For this review, take the finished solid that the model builds, in its own axes (mm). A direction names the side the tool comes from. Coordinates: 2 decimals unless noted, no trailing zeros. Loops run counter-clockwise (first coordinate to the right, second up) from the corner with the lowest first, then second, coordinate; pieces in that order, holes last. Notation, with made-up numbers: (11, -37) -> (34, -37) arc R15 cw to (34, -15) -> close; hole circle Ø5 at (-18, 12.25). An arc over 180 degrees is marked (long way). Answer in a Markdown table with one row per item.
Autodesk Inventor part; units mm, degrees
ref_plane "YZ Plane" through (0, 0, 0) normal (1, 0, 0) x (0, 1, 0)
ref_plane "XZ Plane" through (0, 0, 0) normal (0, 1, 0) x (-1, 0, 0)
ref_plane "XY Plane" through (0, 0, 0) normal (0, 0, 1) x (1, 0, 0)
sketch "Sketch1" plane through (0, 0, 0) normal (0, 0, 1) x (1, 0, 0)
  arc A0 (4.25, 0) -> (-4.25, 0) centre (0, 0) ccw
  line L0 (-18.2, 0) -> (18.2, 0)
  line L1 (-13, 0) -> (-13, 5.25)
  line L2 (-13, 5.25) -> (13, 5.25)
  line L3 (13, 5.25) -> (13, 0)
  line L4 (-13, 0) -> (-4.25, 0)
  line L5 (4.25, 0) -> (13, 0)
  dimension "d0" = 8.5
  dimension "d1" = 1
  dimension "d2" = 13
  dimension "d3" = 13
extrude "Extrusion1" add sketch "Sketch1" along normal blind 20 contours A0 L0 L1 L2 L3
sketch "Sketch2" plane through (-13, 5.25, 0) normal (0, 1, 0) x (1, 0, 0)
  line L0 (-4.8106, -10) -> (24.391, -10) construction
  line L1 (26, 0) -> (0, 0) construction
  line L2 (26, -20) -> (0, -20) construction
  circle A0 centre (5, -10) radius 2.4
  circle A1 centre (21, -10) radius 2.4
  point P0 (13, 0)
  dimension "d7" = 20
  dimension "d8" = 10
  dimension "d9" = 4.8
  dimension "d10" = 4.8
  dimension "d11" = 16
  dimension "d12" = 8
extrude "Extrusion2" cut sketch "Sketch2" against normal through all
sketch "Sketch3" plane through (-13, 0, 0) normal (0, -1, 0) x (1, 0, 0)
  line L0 (0, 0) -> (0, 20)
  line L1 (0, 2) -> (2, 2)
  line L2 (2, 2) -> (2, 18)
  line L3 (2, 18) -> (0, 18)
  line L4 (0, 18) -> (0, 2)
  line L5 (26, 0) -> (26, 20)
  line L6 (26, 2) -> (24, 2)
  line L7 (24, 2) -> (24, 18)
  line L8 (24, 18) -> (26, 18)
  line L9 (26, 18) -> (26, 2)
  line L10 (0, 0) -> (8.75, 0)
  line L11 (0, 20) -> (8.75, 20)
  line L12 (17.25, 20) -> (26, 20)
  line L13 (17.25, 0) -> (26, 0)
  point P0 (13, 0)
  point P1 (0, 18)
  dimension "d15" = 2
  dimension "d16" = 2
  dimension "d17" = 2
  dimension "d18" = 2
  dimension "d19" = 2
  dimension "d20" = 2
extrude "Extrusion3" cut sketch "Sketch3" against normal blind 2
chamfer "Chamfer1" distance 0.5 angle 45 4 edges at (13, 5.25, 10) (0, 5.25, 20) (-13, 5.25, 10) (0, 5.25, 0)
sketch "Sketch4" plane through (0, 0, 20) normal (0, 0, 1) x (1, 0, 0)
  arc A0 (4.25, 0) -> (-4.25, 0) centre (0, 0) ccw
  line L0 (4.25, 0) -> (13, 0)
  line L1 (-13, 0) -> (-4.25, 0)
  line L2 (4.25, 0) -> (-4.25, 0)
extrude "Extrusion4" add sketch "Sketch4" against normal blind 4
equation "\"d8\" = 0.5 * d7"
equation "\"d10\" = d9"
equation "\"d16\" = d15"
equation "\"d17\" = d15"
equation "\"d18\" = d16"
equation "\"d19\" = d16"
equation "\"d20\" = d17"
properties part number "_3DPrint"
Item 1: Take a section at B-B, the plane x = 8. State the section outline as (y, z) points.
Worked answers:
| item | result |
|---|---|
| outline | (0, 0) -> (4.75, 0) -> (5.25, 0.5) -> (5.25, 7.6) -> (0, 7.6) -> close; (0, 12.4) -> (5.25, 12.4) -> (5.25, 19.5) -> (4.75, 20) -> (0, 20) -> close |
Item 2: The part is to be moulded in two halves that separate along Z. For faces 1 (the flat face through (0, 2, 20)), 2 (the flat face through (-13, 3, 10)), 3 (the cylindrical face through (9.29, 2.662, 7.976)), say which applies: +Z half, -Z half, draft (parallel to the pull), parting line (faces both ways), or undercut.
Worked answers:
| item | result |
|---|---|
| face 1 | +Z half |
| face 2 | draft |
| face 3 | undercut |
Item 3: For L1, parallel to Z at x = 8, y = 3.45; L2, parallel to Z at x = -7.5, y = 0.6; L3, parallel to X at y = 1.3, z = 10, list the stretches that pass through material, from the lowest coordinate up.
Worked answers:
| item | result |
|---|---|
| L1 | 0 to 7.6, 12.4 to 20 |
| L2 | 0 to 7.65, 12.35 to 20 |
| L3 | -11 to -10.4, -5.6 to -4.05, 4.05 to 5.6, 10.4 to 11 |
Item 4: Take a section at D-D, the plane z = 2.75. State the section outline as (x, y) points.
Worked answers:
| item | result |
|---|---|
| outline | (-13, 2) -> (-11, 2) -> (-11, 0) -> (-4.25, 0) arc R4.25 cw to (4.25, 0) -> (11, 0) -> (11, 2) -> (13, 2) -> (13, 4.75) -> (12.5, 5.25) -> (-12.5, 5.25) -> (-13, 4.75) -> close |
Item 5: For faces 4 (the cylindrical face through (-0.09, 4.25, 7.89)), 5 (the flat face through (0, 5.25, 10)), 6 (the flat face through (12, 2, 10)), 7 (the cylindrical face through (-10.398, 2.662, 9.894)), 8 (the flat face through (-12, 2, 10)), list the 3-axis set-ups (+Z, -Z, +X, -X, +Y, -Y) from which the entire face can be reached by the end or side of a thin tool; tool diameter is ignored.
Worked answers:
| item | result |
|---|---|
| face 4 | -Z, -Y |
| face 5 | +Z, -Z, +X, -X, +Y |
| face 6 | +X, -Y |
| face 7 | +Y, -Y |
| face 8 | -X, -Y |
Item 6: Take a section at A-A, the plane z = 10. State the section outline as (x, y) points, and give its area (3 significant figures).
Worked answers:
| item | result |
|---|---|
| outline | (-13, 2) -> (-11, 2) -> (-11, 0) -> (-10.4, 0) -> (-10.4, 5.25) -> (-12.5, 5.25) -> (-13, 4.75) -> close; (-5.6, 0) -> (-4.25, 0) arc R4.25 cw to (4.25, 0) -> (5.6, 0) -> (5.6, 5.25) -> (-5.6, 5.25) -> close; (10.4, 0) -> (11, 0) -> (11, 2) -> (13, 2) -> (13, 4.75) -> (12.5, 5.25) -> (10.4, 5.25) -> close |
| area | 49.5 mm² |
Item 7: Take a section at C-C, the plane y = 1.3. State the section outline as (x, z) points.
Worked answers:
| item | result |
|---|---|
| outline | (-13, 0) -> (-4.05, 0) -> (-4.05, 16) -> (4.05, 16) -> (4.05, 0) -> (13, 0) -> (13, 2) -> (11, 2) -> (11, 18) -> (13, 18) -> (13, 20) -> (-13, 20) -> (-13, 18) -> (-11, 18) -> (-11, 2) -> (-13, 2) -> close; hole circle Ø4.8 at (-8, 10); hole circle Ø4.8 at (8, 10) |
Item 8: Insertion check: pin 1 (0.6 mm diameter, centred on y = 1.5, z = 11, fed in from +X); pin 2 (4 mm diameter, centred on x = -8, z = 10, fed in from +Y); pin 3 (1 mm diameter, centred on x = 1, z = 13, fed in from -Y); pin 4 (1.6 mm diameter, centred on x = -12, z = 8, fed in from -Y). Each pin has a flat end and moves straight along its axis. Give the tip position at first contact, or say it passes through.
Worked answers:
| item | result |
|---|---|
| pin 1 | x = 11 |
| pin 2 | through |
| pin 3 | y = 3.98 |
| pin 4 | y = 2 |
